Drawing for the job (mm, zero at the part's lowest x, y, z). Coordinates: 2 decimals unless noted, no trailing zeros. Order: outer loops, then holes, each group sorted by start corner. A loop starts at its lowest first (then second) coordinate and runs counter-clockwise, first axis right, second up. Notation, with made-up numbers: (23.25, 28.5) - (32.25, 28.5) arc R25 cw to (32.25, 52.5) - close; hole circle Ø6 at (82.25, 80). An arc over 180 degrees is marked (long way). Put each result on its own line as item: value. Start each with the question number.
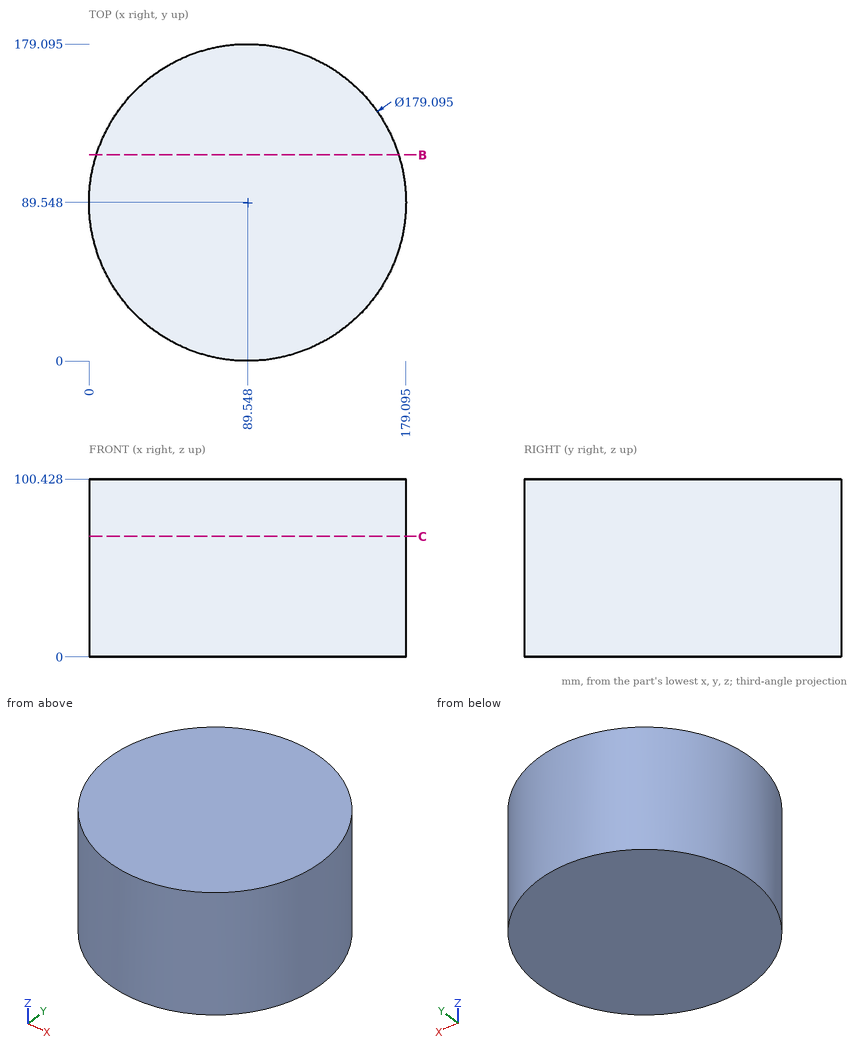
Item 1: Slice it at C-C, the plane z = 68. Give the cut face in (x, y) (1 decimal).
Item 2: Wall check: line 1 along X through (y, z) = (92, 46.5); line 2 along X through (y, z) = (143, 14) (1 decimal); line 3 along Y through (x, z) = (79, 11). Give the ranges that are in metal, low to high.
Item 3: Slice it at B-B, the plane y = 116.5. Give the cut face in (x, z).
Item 4: Flat gauge pins, fed straight in: pin 1 Ø10 at (x, y) = (149.5, 21.5) entering from +Z; pin 2 Ø1.5 at (x, z) = (34.5, 71.5) entering from -Y; pin 3 Ø8 at (y, z) = (110, 87) entering from +X; pin 4 Ø1.5 at (x, z) = (19.5, 86.5) entering from +Y (1 decimal). Where does each tip first touch, or does it go through?
Here are the results:
1. outline: circle Ø179.1 at (89.5, 89.5)
2. line 1: x = 0.03 to 179.06
2. line 2: x = 17.7 to 161.4
2. line 3: y = 0.62 to 178.47
3. outline: (4.15, 0) - (174.94, 0) - (174.94, 100.43) - (4.15, 100.43) - close
4. pin 1: stops at z = 100.43
4. pin 2: stops at y = 18.34
4. pin 3: stops at x = 177.57
4. pin 4: stops at y = 146.3
